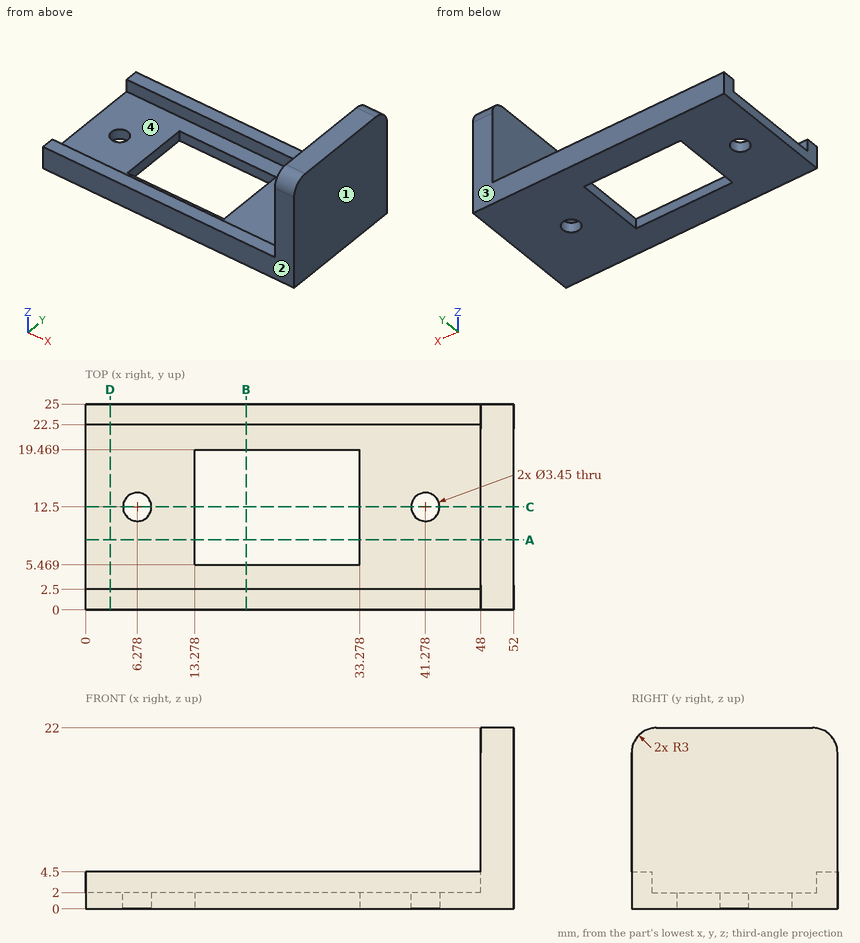
For this review, use the dimensioned drawing (mm, ordinates from the lowest corner) and the shaded views. Give positions to 0.01 mm unless a question says otherwise; leave off trailing zeros. Loops run counter-clockwise (first coordinate to the right, second up) from the corner with the lowest first, then second, coordinate; pieces in that order, holes last.
Item 1: For line 1 along Z through (x, y) = (13, 18.75); line 2 along X through (y, z) = (6.75, 20.25); line 3 along Y through (x, z) = (42.5, 1), list the stretches that pass through material, from the lowest coordinate up.
Item 2: Take a section at D-D, the plane x = 3. State the section outline as (y, z) points, and give its area (3 significant figures).
Item 3: Draft analysis for pull direction Y (two halves, no side actions). For the marked faces 1, 2, 3 and 4, state which applies: +Y half, -Y half, draft (parallel to the pull), parting line (faces both ways), or undercut.
Item 4: Take a section at C-C, the plane y = 12.5. State the section outline as (x, z) points.
Item 5: Take a section at A-A, the plane y = 8.5. State the section outline as (x, z) points.
Item 6: Insertion check: pin 1 (3 mm diameter, centred on x = 21.5, y = 1.5, fed in from +Z); pin 2 (1.5 mm diameter, centred on x = 32, z = 7, fed in from +Y); pin 3 (1 mm diameter, centred on y = 11, z = 13, fed in from -X). Each pin has a flat end and moves straight along its axis. Give the tip position at first contact, or say it passes through.
Item 7: Take a section at B-B, the plane x = 19.5. State the section outline as (y, z) points.
Calculated:
1. line 1: z = 0 to 2
1. line 2: x = 48 to 52
1. line 3: y = 0 to 11.28, 13.72 to 25
2. outline: (0, 0) - (25, 0) - (25, 4.5) - (22.5, 4.5) - (22.5, 2) - (2.5, 2) - (2.5, 4.5) - (0, 4.5) - close
2. area: 62.5 mm2
3. face 1: draft
3. face 2: -Y half
3. face 3: +Y half
3. face 4: undercut
4. outline: (0, 0) - (4.55, 0) - (4.55, 2) - (0, 2) - close; (8, 0) - (13.28, 0) - (13.28, 2) - (8, 2) - close; (33.28, 0) - (39.55, 0) - (39.55, 2) - (33.28, 2) - close; (43, 0) - (52, 0) - (52, 22) - (48, 22) - (48, 2) - (43, 2) - close
5. outline: (0, 0) - (13.28, 0) - (13.28, 2) - (0, 2) - close; (33.28, 0) - (52, 0) - (52, 22) - (48, 22) - (48, 2) - (33.28, 2) - close
6. pin 1: stops at z = 4.5
6. pin 2: passes through
6. pin 3: stops at x = 48
7. outline: (0, 0) - (5.47, 0) - (5.47, 2) - (2.5, 2) - (2.5, 4.5) - (0, 4.5) - close; (19.47, 0) - (25, 0) - (25, 4.5) - (22.5, 4.5) - (22.5, 2) - (19.47, 2) - close
